from build123d import *

# Parameters (mm, degrees)
SKETCH1_R           = 25
SKETCH1_R_2         = 15
BOSS_EXTRUDE1_DEPTH = 25
BOSS_EXTRUDE2_START = -30
BOSS_EXTRUDE2_DEPTH = 10
BOSS_EXTRUDE3_START = 15
BOSS_EXTRUDE3_DEPTH = 9
HOLE1_D             = 12


with BuildPart() as part:
    # Sketch1 → Boss-Extrude1 (new, symmetric)
    with BuildSketch(Plane.XY):
        Circle(SKETCH1_R)
        Circle(SKETCH1_R_2, mode=Mode.SUBTRACT)
    extrude(amount=BOSS_EXTRUDE1_DEPTH, both=True)

    # Sketch3 → Boss-Extrude2 (add)
    with BuildSketch(Plane(origin=(0, 0, -25), x_dir=(-1, 0, 0), z_dir=(0, 0, -1)).offset(BOSS_EXTRUDE2_START)):
        with BuildLine():
            Line((-104, 15), (-104, -15))
            Line((-104, -15), (-2.420790466, -24.882519437))
            ThreePointArc((-2.420790466, -24.882519437), (-25, 0), (-2.420790466, 24.882519437))
            Line((-2.420790466, 24.882519437), (-104, 15))
        make_face()
    extrude(amount=BOSS_EXTRUDE2_DEPTH)

    # Sketch6 → Boss-Extrude3 (add)
    with BuildSketch(Plane(origin=(0, 0, 0), x_dir=(1, 0, 0), z_dir=(0, 1, 0)).offset(BOSS_EXTRUDE3_START)):
        with BuildLine():
            Line((104, -5), (104, 20))
            ThreePointArc((104, 20), (116, 32), (128, 20))
            Line((128, 20), (128, -5))
            Line((128, -5), (104, -5))
        make_face()
    boss_extrude3 = extrude(amount=-BOSS_EXTRUDE3_DEPTH)

    # Mirror1: Boss-Extrude3 across plane
    add(boss_extrude3.mirror(Plane.ZX))

    # Hole1 (through all)
    with Locations(Plane(origin=(0, 15, 0), x_dir=(1, 0, 0), z_dir=(0, 1, 0))):
        with Locations((116, 20)):
            Hole(HOLE1_D / 2)


solid = part.part
Geometry check sheet. Reference: the model listing, model coordinates, mm. A direction names the side the tool comes from. Give positions to 0.01 mm unless a question says otherwise; leave off trailing zeros. Order: outer loops, then holes, each group sorted by start corner. A loop starts at its lowest first (then second) coordinate and runs counter-clockwise, first axis right, second up. Notation, with made-up numbers: M 83,30.5 L 106,30.5 A27 ccw 106,58.5 Z; hole C 49.5,34 d2. An arc over 180 degrees is marked long. Use a Markdown table: item, result.
Item 1: Section check C-C (z = 3). Record the cut outline in (x, y), and give its area (3 significant figures).
Answers follow:
| item | result |
|---|---|
| outline | M 2.42,-24.88 L 104,-15 L 128,-15 L 128,-6 L 104,-6 L 104,6 L 128,6 L 128,15 L 104,15 L 2.42,24.88 A25 ccw long Z; hole C 0,0 d30 |
| area | 4,880 mm2 |
Item 2: Depth check by flat-ended pin: P1, Ø4, axis at x = -9.5, z = 2, coming from the +Y side; P2, Ø7, axis at x = 116, z = -20, coming from the +Y side; P3, Ø7, axis at x = 117.5, z = -17, coming from the -Y side; P4, Ø1, axis at x = 97, y = -9.5, coming from the -Z side. Enter the tip coordinate at first touch or a pass-through.
Answers follow:
| item | result |
|---|---|
| P1 | stops at y = 23.85 |
| P2 | passes through |
| P3 | stops at y = -15 |
| P4 | stops at z = -5 |
Item 3: Section check A-A (y = 0). Record the cut outline in (x, z), and give its area (3 significant figures).
Answers follow:
| item | result |
|---|---|
| outline | M -25,-25 L -15,-25 L -15,25 L -25,25 Z; M 15,-25 L 25,-25 L 25,-5 L 104,-5 L 104,5 L 25,5 L 25,25 L 15,25 Z |
| area | 1,790 mm2 |
Item 4: Material ranges on line 1 along Y through (x, z) = (114, -28.5); line 2 along X through (y, z) = (-9, -20); line 3 along X through (y, z) = (-10, -21), recorded low to high.
Answers follow:
| item | result |
|---|---|
| line 1 | y = -15 to -6, 6 to 15 |
| line 2 | x = -23.32 to -12, 12 to 23.32, 104 to 110, 122 to 128 |
| line 3 | x = -22.91 to -11.18, 11.18 to 22.91, 104.04 to 110.08, 121.92 to 127.96 |
Item 5: Draft check along Y on faces 4 (the cylindrical face through (-24.976, 1.099, 0.35)), 5 (the cylindrical face through (-14.985, 0.66, -0.35)), 6 (the flat face through (104, 11, -12)), 7 (the flat face through (116, 6, -10)). Enter one of: +Y half, -Y half, draft (parallel to the pull), parting line (faces both ways), or undercut.
Answers follow:
| item | result |
|---|---|
| face 4 | parting line |
| face 5 | undercut |
| face 6 | draft |
| face 7 | undercut |
Item 6: Tool access check on faces 1 (the flat face through (116, 15, -10)), 2 (the flat face through (104, -11, -12)), 3 (the flat face through (116, -15, -10)). Record the directions out of +Z, -Z, +X, -X, +Y, -Y that give a thin tool (end or side, any length) a straight path to the whole face; none if there is none.
Answers follow:
| item | result |
|---|---|
| face 1 | +Z, -Z, +X, +Y |
| face 2 | -Z, +Y, -Y |
| face 3 | +Z, -Z, +X, -Y |
Item 7: Section check D-D (x = 116). Record the cut outline in (y, z).
Answers follow:
| item | result |
|---|---|
| outline | M -15,-32 L -6,-32 L -6,-26 L -15,-26 Z; M -15,-14 L -6,-14 L -6,5 L -15,5 Z; M 6,-32 L 15,-32 L 15,-26 L 6,-26 Z; M 6,-14 L 15,-14 L 15,5 L 6,5 Z |
Item 8: Section check B-B (x = 0). Record the cut outline in (y, z), and give its area (3 significant figures).
Answers follow:
| item | result |
|---|---|
| outline | M -25,-25 L -15,-25 L -15,25 L -25,25 Z; M 15,-25 L 25,-25 L 25,25 L 15,25 Z |
| area | 1,000 mm2 |
